The drawing under review shows one solid part. Ordinate dimensions are in mm from its lowest x, y, z. A direction names the side the tool comes from. Coordinates: 2 decimals unless noted, no trailing zeros. Loops run counter-clockwise (first coordinate to the right, second up) from the corner with the lowest first, then second, coordinate; pieces in that order, holes last. Notation, with made-up numbers: M 74.5,-35.5 L 95.5,-35.5 A27 ccw 95.5,-6.5 Z; hole C 55.25,76.5 d1. An arc over 180 degrees is marked long. Answer as a JSON object with one key per item and string values. Group by question number.
1. Consider section A-A (x = 2.75). State the section outline as (y, z) points.
2. Consider section B-B (y = 2.75). State the section outline as (x, z) points.
3. To check wall thickness, follow probe 1 along Z at (x, y) = (1.55, 1.3); probe 2 along Y at (x, z) = (2.85, 4.75); probe 3 along Y at (x, z) = (3.4, 11.75). State the ranges of each line that lie inside material, in increasing order.
4. Consider section C-C (z = 10.5). State the section outline as (x, y) points.
5. Machinability: for the marked faces 1 and 2, which of the approach directions +Z, -Z, +X, -X, +Y, -Y give a long, thin tool a straight path to every point of the face, cutting with its end or side? Answer none if there is none.
6. Insertion check: pin 1 (1 mm diameter, centred on y = 2.5, z = 4.5, fed in from +X); pin 2 (0.6 mm diameter, centred on x = 2, z = 0, fed in from +Y); pin 3 (1 mm diameter, centred on y = 4, z = 3.5, fed in from +X). Each pin has a flat end and moves straight along its axis. Give the tip position at first contact, or say it passes through.
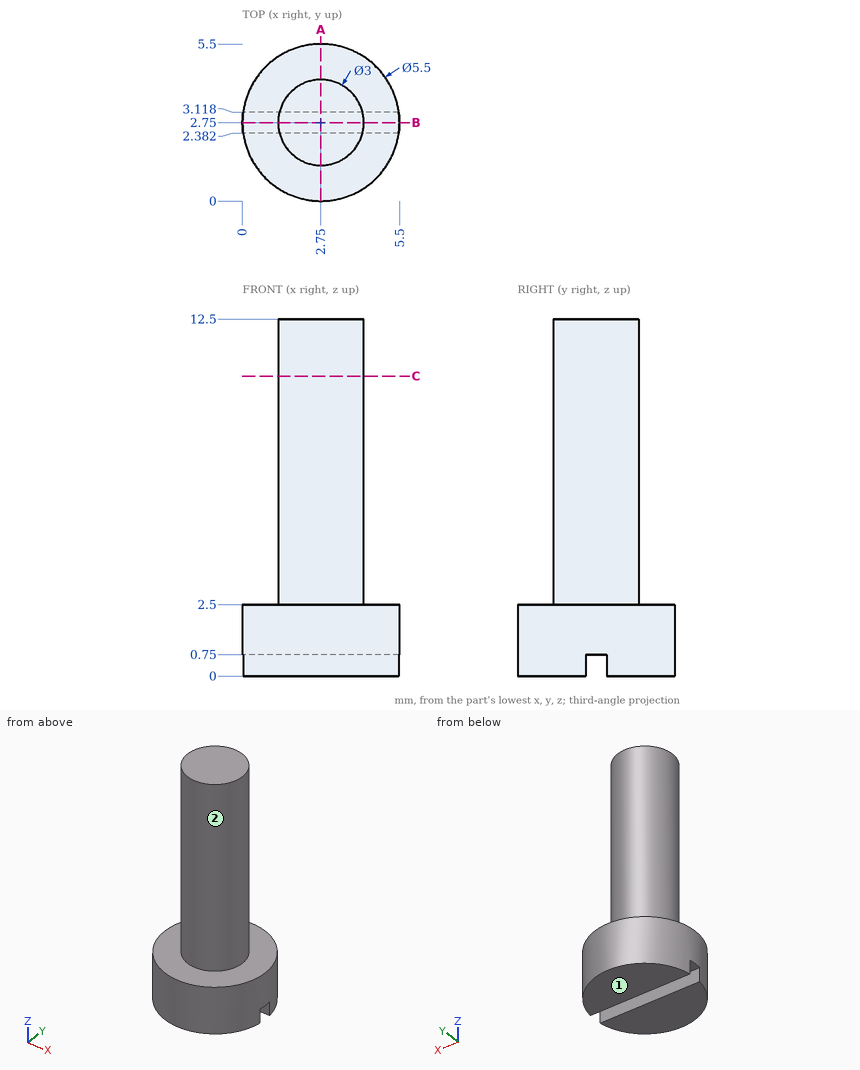
Findings below:
{
 "1": {"outline": "M 0,0 L 2.38,0 L 2.38,0.75 L 3.12,0.75 L 3.12,0 L 5.5,0 L 5.5,2.5 L 4.25,2.5 L 4.25,12.5 L 1.25,12.5 L 1.25,2.5 L 0,2.5 Z"},
 "2": {"outline": "M 0,0.75 L 5.5,0.75 L 5.5,2.5 L 4.25,2.5 L 4.25,12.5 L 1.25,12.5 L 1.25,2.5 L 0,2.5 Z"},
 "3": {"probe 1": "z = 0 to 2.5", "probe 2": "y = 1.25 to 4.25", "probe 3": "y = 1.4 to 4.1"},
 "4": {"outline": "C 2.75,2.75 d3"},
 "5": {"face 1": "-Z, +X, -X, +Y, -Y", "face 2": "+Z"},
 "6": {"pin 1": "stops at x = 4.25", "pin 2": "stops at y = 5.46", "pin 3": "stops at x = 4.05"}
}
